Input: part model. Units: mm. Frame: model coordinates. Give positions to 0.01 mm unless a question says otherwise; leave off trailing zeros. Write each loop counter-clockwise with the first axis right and the second up, starting at its lowest first coordinate (ties: lowest second). Pieces come first, ordered by that corner, then holes.
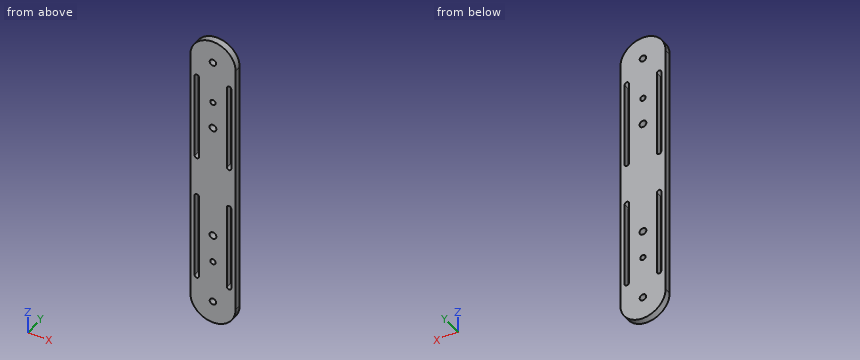
```python
from build123d import *

# Parameters (mm, degrees)
SKETCH1_R               = 1.5
BOSS_EXTRUDE1_DEPTH     = 3.175
CUT_EXTRUDE1_DEPTH      = 131.960225355
CUT_EXTRUDE1_DEPTH_BACK = 131.960225355
CUT_EXTRUDE2_DEPTH      = 131.960225355
CUT_EXTRUDE2_DEPTH_BACK = 131.960225355
CUT_EXTRUDE3_DEPTH      = 131.960225355
CUT_EXTRUDE3_DEPTH_BACK = 131.960225355
SKETCH4_R               = 1.6
CUT_EXTRUDE4_DEPTH      = 40


with BuildPart() as part:
    # Sketch1 → Boss-Extrude1 (new body)
    with BuildSketch(Plane(origin=(0, 0, 0), x_dir=(1, 0, 0), z_dir=(0, 1, 0))):
        with BuildLine():
            Line((-10.5, 0), (-10.5, -120))
            ThreePointArc((-10.5, -120), (0, -130.5), (10.5, -120))
            Line((10.5, -120), (10.5, 0))
            ThreePointArc((10.5, 0), (0, 10.5), (-10.5, 0))
        make_face()
        with Locations(Location((0, 0, 0), (0, 0, 270))):
            Circle(SKETCH1_R, mode=Mode.SUBTRACT)
        with Locations(Location((0, -120, 0), (0, 0, 270))):
            Circle(SKETCH1_R, mode=Mode.SUBTRACT)
    extrude(amount=BOSS_EXTRUDE1_DEPTH)

    # Sketch2 → Cut-Extrude1 (cut, two sides: drawn at the far end of the back side and taken through both)
    with BuildSketch(Plane.XZ.offset(-CUT_EXTRUDE1_DEPTH_BACK)):
        with BuildLine():
            ThreePointArc((0, 18.75), (1.25, 20), (0, 21.25))
            ThreePointArc((0, 21.25), (-1.25, 20), (0, 18.75))
        make_face()
    extrude(amount=CUT_EXTRUDE1_DEPTH + CUT_EXTRUDE1_DEPTH_BACK, mode=Mode.SUBTRACT)

    # Sketch3 → Cut-Extrude2 (cut, two sides: drawn at the far end of the back side and taken through both)
    with BuildSketch(Plane(origin=(0, 3.175, 0), x_dir=(1, 0, 0), z_dir=(0, 1, 0)).offset(-CUT_EXTRUDE2_DEPTH_BACK)):
        with BuildLine():
            ThreePointArc((0, -98.75), (-1.25, -100), (0, -101.25))
            ThreePointArc((0, -101.25), (1.25, -100), (0, -98.75))
        make_face()
    extrude(amount=CUT_EXTRUDE2_DEPTH + CUT_EXTRUDE2_DEPTH_BACK, mode=Mode.SUBTRACT)

    # Sketch4 → Cut-Extrude3 (cut, two sides: drawn at the far end of the back side and taken through both)
    with BuildSketch(Plane(origin=(0, 3.175, 0), x_dir=(1, 0, 0), z_dir=(0, 1, 0)).offset(-CUT_EXTRUDE3_DEPTH_BACK)):
        with Locations(Location((0, -33.15, 0), (0, 0, 270))):
            Circle(SKETCH4_R)
        with Locations(Location((0, -87.15, 0), (0, 0, 270))):
            Circle(SKETCH4_R)
    extrude(amount=CUT_EXTRUDE3_DEPTH + CUT_EXTRUDE3_DEPTH_BACK, mode=Mode.SUBTRACT)

    # Sketch5 → Cut-Extrude4 (cut)
    with BuildSketch(Plane.XZ):
        with BuildLine():
            Line((-8.5, 10), (-8.5, 50))
            ThreePointArc((-8.5, 50), (-7.5, 51), (-6.5, 50))
            Line((-6.5, 50), (-6.5, 10))
            ThreePointArc((-6.5, 10), (-7.5, 9), (-8.5, 10))
        make_face()
        with BuildLine():
            Line((6.5, 50), (6.5, 10))
            ThreePointArc((6.5, 10), (7.5, 9), (8.5, 10))
            Line((8.5, 10), (8.5, 50))
            ThreePointArc((8.5, 50), (7.5, 51), (6.5, 50))
        make_face()
        with BuildLine():
            Line((8.5, 110), (8.5, 70))
            ThreePointArc((8.5, 70), (7.5, 69), (6.5, 70))
            Line((6.5, 70), (6.5, 110))
            ThreePointArc((6.5, 110), (7.5, 111), (8.5, 110))
        make_face()
        with BuildLine():
            Line((-6.5, 70), (-6.5, 110))
            ThreePointArc((-6.5, 110), (-7.5, 111), (-8.5, 110))
            Line((-8.5, 110), (-8.5, 70))
            ThreePointArc((-8.5, 70), (-7.5, 69), (-6.5, 70))
        make_face()
    extrude(amount=-CUT_EXTRUDE4_DEPTH, mode=Mode.SUBTRACT)


solid = part.part
```
Q1. Section A-A, the plane z = 74. Return the cut outline in (x, y) (3 decimals), then the cut area to 3 significant figures.
Q2. Pin query (flat end, axial travel): pin 1 (1.9 mm diameter, centred on x = 0, z = 87.15, fed in from +Y). Return the tip coordinate at first contact, or that it passes through.
Q3. Material intervals for line 1 along X through (y, z) = (1.55, 96); line 2 along X through (y, z) = (1.35, 100); line 3 along X through (y, z) = (1, 33.15), sorted ascending.
Q4. Section B-B, the plane y = 2.4. Give the number of separate pieces and of enclosed holes in the cut face, then the cut area to 3 significant figures.
Solutions:
1. outline: (-10.5, 0) - (-8.5, 0) - (-8.5, 3.175) - (-10.5, 3.175) - close; (-6.5, 0) - (6.5, 0) - (6.5, 3.175) - (-6.5, 3.175) - close; (8.5, 0) - (10.5, 0) - (10.5, 3.175) - (8.5, 3.175) - close
1. area: 54.0 mm2
2. pin 1: passes through
3. line 1: x = -10.5 to -8.5, -6.5 to 6.5, 8.5 to 10.5
3. line 2: x = -10.5 to -8.5, -6.5 to -1.25, 1.25 to 6.5, 8.5 to 10.5
3. line 3: x = -10.5 to -8.5, -6.5 to -1.6, 1.6 to 6.5, 8.5 to 10.5
4. separate pieces: 1
4. enclosed holes: 10
4. area: 2,490 mm2
